Read the model definition and answer for the solid it produces. Units are mm, in the model's axes. Coordinates: 2 decimals unless noted, no trailing zeros. Order: outer loops, then holes, each group sorted by start corner. A loop starts at its lowest first (then second) coordinate and runs counter-clockwise, first axis right, second up. Notation, with made-up numbers: (58.5, 51) - (81.5, 51) arc R31 ccw to (81.5, 76) - close; hole circle Ø11 at (85, 70). An arc over 180 degrees is marked (long way). Write item = value, one per line.
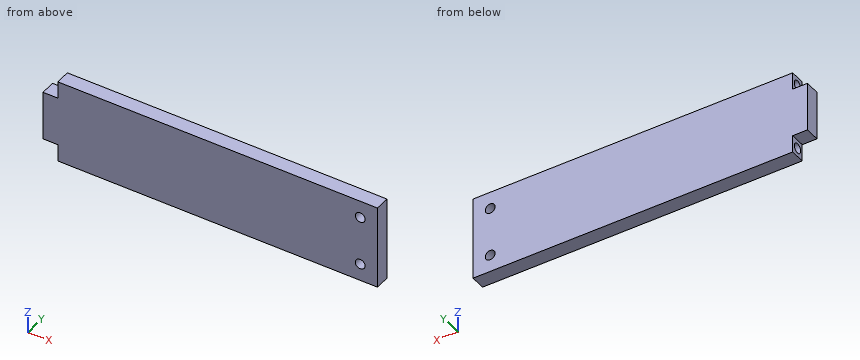
from build123d import *

# Parameters (mm, degrees)
BOSS_EXTRU_1_DEPTH      = 6
ESQUISSE3_R             = 2
ENL_V_MAT_EXTRU_2_DEPTH = 10
ESQUISSE5_R             = 2
ENL_V_MAT_EXTRU_3_DEPTH = 355.348418967


with BuildPart() as part:
    # Esquisse2 → Boss.-Extru.1 (new body)
    with BuildSketch(Plane(origin=(0, 0, 0), x_dir=(1, 0, 0), z_dir=(0, 1, 0))):
        Polygon((-347.889533646, 17), (-217.889533646, 17), (-217.889533646, -17), (-347.889533646, -17), (-347.889533646, -10), (-353.889533646, -10), (-353.889533646, 10), (-347.889533646, 10), align=None)
    extrude(amount=BOSS_EXTRU_1_DEPTH)

    # Esquisse3 → Enlèv. mat.-Extru.2 (cut)
    with BuildSketch(Plane.ZY.offset(347.889533646)):
        with Locations((-13.5, 3)):
            Circle(ESQUISSE3_R)
        with Locations((13.5, 3)):
            Circle(ESQUISSE3_R)
    extrude(amount=-ENL_V_MAT_EXTRU_2_DEPTH, mode=Mode.SUBTRACT)

    # Esquisse5 → Enlèv. mat.-Extru.3 (cut, through all)
    with BuildSketch(Plane(origin=(0, 6, 0), x_dir=(1, 0, 0), z_dir=(0, 1, 0))):
        with Locations(Location((-224.889533646, 10, 0), (0, 0, 270))):
            Circle(ESQUISSE5_R)
        with Locations(Location((-224.889533646, -10, 0), (0, 0, 90))):
            Circle(ESQUISSE5_R)
    extrude(amount=-ENL_V_MAT_EXTRU_3_DEPTH, mode=Mode.SUBTRACT)


solid = part.part
1) The part is cut by section A-A (z = -13.5). Determine the outline of the cut face in (x, y).
Returned:
outline = (-347.89, 0) - (-217.89, 0) - (-217.89, 6) - (-347.89, 6) - (-347.89, 5) - (-337.89, 5) - (-337.89, 1) - (-347.89, 1) - close
2) Flat-ended cylindrical pins translate along their axes: pin 1 Ø2.5 at (x, z) = (-224.89, -10) entering from -Y; pin 2 Ø2 at (y, z) = (3, 13.5) entering from -X; pin 3 Ø3 at (x, y) = (-351, 2.5) entering from -Z; pin 4 Ø2 at (y, z) = (2.5, -14.5) entering from -X. Find the tip coordinate at first contact, or state that the pin passes through.
Returned:
pin_1 = through
pin_2 = -337.89
pin_3 = -10
pin_4 = -347.89
3) The part is cut by section B-B (y = 2). Determine the outline of the cut face in (x, z), and give its area (3 significant figures).
Returned:
outline = (-353.89, -10) - (-347.89, -10) - (-347.89, -11.77) - (-337.89, -11.77) - (-337.89, -15.23) - (-347.89, -15.23) - (-347.89, -17) - (-217.89, -17) - (-217.89, 17) - (-347.89, 17) - (-347.89, 15.23) - (-337.89, 15.23) - (-337.89, 11.77) - (-347.89, 11.77) - (-347.89, 10) - (-353.89, 10) - close; hole circle Ø4 at (-224.89, -10); hole circle Ø4 at (-224.89, 10)
area = 4,450 mm^2
4) Straight lines are drawn through the part: line 1 along Y through (x, z) = (-345.25, -13.5); line 2 along Y through (x, z) = (-340, 13); line 3 along X through (y, z) = (4.3, -14). For each, find the intervals that lie inside material, in ascending order. Write a range as from..to.
Returned:
line_1 = 0..1, 5..6
line_2 = 0..1.06, 4.94..6
line_3 = -337.89..-217.89
